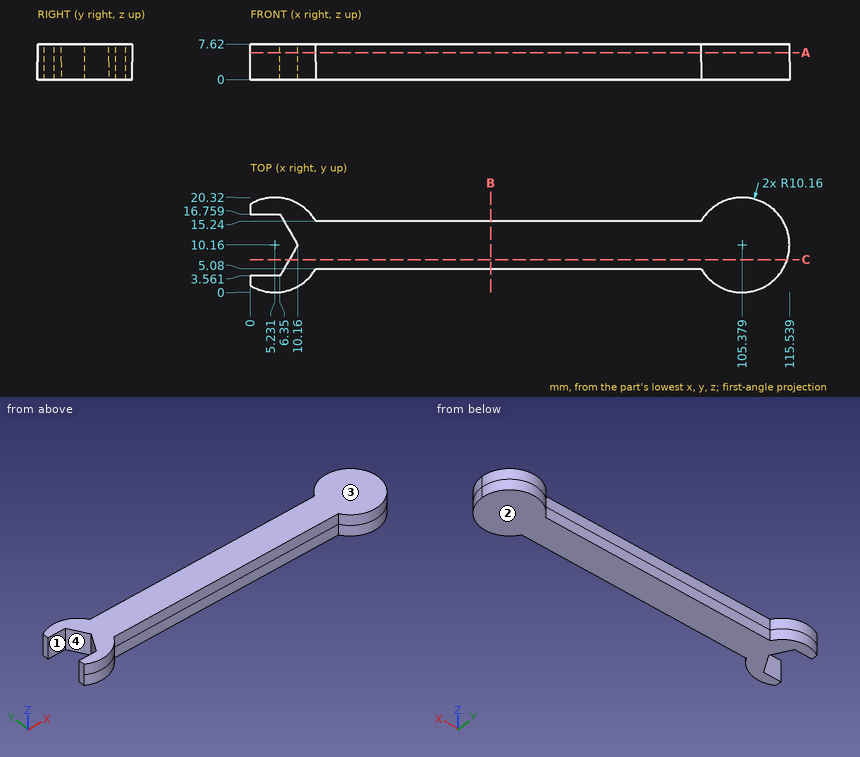
Could you check a few things on this drawing? It's one solid part, dimensions in mm from its lowest x, y, z. A direction names the side the tool comes from. Coordinates: 2 decimals unless noted, no trailing zeros. Order: outer loops, then holes, each group sorted by start corner. A loop starts at its lowest first (then second) coordinate and runs counter-clockwise, first axis right, second up. Notation, with made-up numbers: (11.25, 52.25) - (65.25, 52.25) arc R25 ccw to (65.25, 91.25) - close; hole circle Ø11 at (84, -40). An arc over 180 degrees is marked (long way). One line per question, with ' | ' between items.
(1) If I drill on L1, parallel to Y at x = 71, z = 2.25; L2, parallel to X at y = 17, z = 0.5 (1 decimal); L3, parallel to X at y = 3.75, z = 5.5 (1 decimal), over which ranges is the centre line in solid material (lowest first)?
Report:
L1: y = 5.08 to 15.24 | L2: x = 0 to 12.7, 97.9 to 112.9 | L3: x = 6.5 to 13.1, 97.5 to 113.3
(2) Suppose I cut it at A-A on z = 5.75. List the corners of the cut face in (x, y) for me, and give its area (3 significant figures).
Report:
outline: (0, 1.45) arc R10.16 ccw to (14.03, 5.08) - (96.58, 5.08) arc R10.16 ccw (long way) to (96.58, 15.24) - (14.03, 15.24) arc R10.16 ccw to (0, 18.87) - (0, 16.76) - (6.35, 16.76) - (10.16, 10.16) - (6.35, 3.56) - (0, 3.56) - close | area: 1,300 mm2
(3) Will these pins go through, and if not, where does the flat tip stop? pin 1 (1.1 mm diameter, centred on x = 66.5, z = 5, fed in from +Y); pin 2 (4 mm diameter, centred on x = 92, z = 3.5, fed in from -Y); pin 3 (1 mm diameter, centred on x = 92, y = 17, fed in from +Z).
Report:
pin 1: stops at y = 15.24 | pin 2: stops at y = 5.08 | pin 3: passes through
(4) Suppose I cut it at C-C on y = 7. List the corners of the cut face in (x, z) for me (1 decimal).
Report:
outline: (8.3, 0) - (115, 0) - (115, 7.6) - (8.3, 7.6) - close
(5) For the marked faces 3 and 4, which set-ups out of +Z, -Z, +X, -X, +Y, -Y let a thin tool reach every point of the face, with its end or its side?
Report:
face 3: +Z, +X, -X, +Y, -Y | face 4: +Z, -Z, -X
(6) Suppose I cut it at B-B on x = 51.5. List the corners of the cut face in (y, z) for me.
Report:
outline: (5.08, 0) - (15.24, 0) - (15.24, 7.62) - (5.08, 7.62) - close
(7) If we mould it in two halves opening along Y, with no side actions, what happens to the marked faces 1 and 2? For each: pulls with the +Y half, pulls with the -Y half, needs draft (parallel to the pull), parting line crosses it, or undercut.
Report:
face 1: undercut | face 2: needs draft
